```python
from build123d import *

# Parameters (mm, degrees)
PAD_DEPTH    = 25
SKETCH003_R  = 2.1
POCKET_DEPTH = 25.001


with BuildPart() as part:
    # Sketch → Pad (new body)
    with BuildSketch(Plane.XY):
        Polygon((17, -30), (-20, -30), (-20, 20), (20, 20), (20, 0), (17, 0), align=None)
    extrude(amount=PAD_DEPTH)

    # Sketch003 (on Face8 of Pad) → Pocket (cut, through all)
    with BuildSketch(Plane.XY.offset(25)):
        with Locations((0, -17)):
            Circle(SKETCH003_R)
        with Locations((-11, 0)):
            Circle(SKETCH003_R)
        with Locations((-14, 14)):
            Circle(SKETCH003_R)
        with Locations((14, 14)):
            Circle(SKETCH003_R)
        with Locations((0, 14)):
            Circle(SKETCH003_R)
    extrude(amount=-POCKET_DEPTH, mode=Mode.SUBTRACT)


solid = part.part
```
For this review, take the finished solid that the model builds, in its own axes (mm). A direction names the side the tool comes from. Give positions to 0.01 mm unless a question says otherwise; leave off trailing zeros. Write each loop counter-clockwise with the first axis right and the second up, starting at its lowest first coordinate (ties: lowest second). Pieces come first, ordered by that corner, then holes. Notation, with made-up numbers: M 7,70.25 L 58,70.25 A28 ccw 58,91.25 Z; hole C 38,-35.75 d5. An arc over 180 degrees is marked long. Answer as a JSON object with one key per item and string values. Group by question number.
Item 1: Consider section D-D on x = -14. Write out the cut boundary in (y, z).
Item 2: Consider section B-B on y = 14. Write out the cut boundary in (x, z), plus the area to 3 significant figures.
Item 3: For probe 1 along Y at (x, z) = (0, 9.75); probe 2 along Y at (x, z) = (14, 11.25); probe 3 along X at (y, z) = (-7, 1.5), list the stretches that pass through material, from the lowest coordinate up. Write a range as [from, to].
Item 4: Draft analysis for pull direction X (two halves, no side actions). For faces 1 (the cylindrical face through (11.9, 14.09, 12.68)), 2 (the flat face through (0, -5, 25)), 3 (the cylindrical face through (-13.1, 0.09, 12.68)), 4 (the flat face through (17, -15, 12)), state which applies: +X half, -X half, draft (parallel to the pull), parting line (faces both ways), or undercut.
Item 5: Consider section A-A on x = 0. Write out the cut boundary in (y, z), plus the area to 3 significant figures.
Item 6: Tool access review of faces 5 (the flat face through (0, 20, 12)), 6 (the flat face through (19, 0, 12)): name each direction out of +Z, -Z, +X, -X, +Y, -Y from which nothing blocks a thin tool from reaching the whole face with its end or side.
Item 7: Consider section C-C on z = 10. Write out the cut boundary in (x, y), plus the area to 3 significant figures.
Item 8: For pin 1 Ø1 at (y, z) = (-22, 19) entering from +X; pin 2 Ø0.9 at (x, z) = (18.5, 17.5) entering from -Y, all flat-tipped, find the tip position at first contact; note any pin that passes through.
Check result:
{
 "1": {"outline": "M -30,0 L 11.9,0 L 11.9,25 L -30,25 Z; M 16.1,0 L 20,0 L 20,25 L 16.1,25 Z"},
 "2": {"outline": "M -20,0 L -16.1,0 L -16.1,25 L -20,25 Z; M -11.9,0 L -2.1,0 L -2.1,25 L -11.9,25 Z; M 2.1,0 L 11.9,0 L 11.9,25 L 2.1,25 Z; M 16.1,0 L 20,0 L 20,25 L 16.1,25 Z", "area": "685 mm^2"},
 "3": {"probe 1": "y = [-30, -19.1], [-14.9, 11.9], [16.1, 20]", "probe 2": "y = [-30, 11.9], [16.1, 20]", "probe 3": "x = [-20, 17]"},
 "4": {"face 1": "undercut", "face 2": "draft", "face 3": "undercut", "face 4": "+X half"},
 "5": {"outline": "M -30,0 L -19.1,0 L -19.1,25 L -30,25 Z; M -14.9,0 L 11.9,0 L 11.9,25 L -14.9,25 Z; M 16.1,0 L 20,0 L 20,25 L 16.1,25 Z", "area": "1,040 mm^2"},
 "6": {"face 5": "+Z, -Z, +X, -X, +Y", "face 6": "+Z, -Z, +X, -Y"},
 "7": {"outline": "M -20,-30 L 17,-30 L 17,0 L 20,0 L 20,20 L -20,20 Z; hole C -14,14 d4.2; hole C -11,0 d4.2; hole C 0,-17 d4.2; hole C 0,14 d4.2; hole C 14,14 d4.2", "area": "1,840 mm^2"},
 "8": {"pin 1": "stops at x = 17", "pin 2": "stops at y = 0"}
}
